Autodesk Inventor part; units mm, degrees
ref_plane "rail25_to_dummy_XY" through (0, 0, 320) normal (0, 0, 1) x (1, 0, 0)
ref_plane "rail25_to_dummy_YZ" through (0, 0, 320) normal (1, 0, 0) x (0, 1, 0)
ref_plane "rail25_to_dummy_ZX" through (0, 0, 320) normal (0, 1, 0) x (0, 0, 1)
sketch "Sketch_1" plane through (0, 0, 0) normal (0, 0, 1) x (1, 0, 0)
  arc A0 (-12.5, 1) -> (-11.5, 0) centre (-11.5, 1) ccw
  line L0 (-11.5, 0) -> (11.5, 0)
  arc A1 (11.5, 0) -> (12.5, 1) centre (11.5, 1) ccw
  line L1 (12.5, 1) -> (12.5, 7.5)
  arc A2 (12.5, 7.5) -> (11.5, 8.5) centre (11.5, 7.5) ccw
  line L2 (11.5, 8.5) -> (9.5, 8.5)
  arc A3 (9.5, 8.5) -> (8.6036, 7.9432) centre (9.5, 7.5) ccw
  arc A4 (8.5, 3.4087) -> (8.6036, 7.9432) centre (7.5, 5.7) ccw
  line L3 (8.5, 3.4087) -> (8.5, 2.5)
  arc A5 (8, 2) -> (8.5, 2.5) centre (8, 2.5) ccw
  line L4 (8, 2) -> (-8, 2)
  arc A6 (-8.5, 2.5) -> (-8, 2) centre (-8, 2.5) ccw
  line L5 (-8.5, 2.5) -> (-8.5, 3.4087)
  arc A7 (-8.6036, 7.9432) -> (-8.5, 3.4087) centre (-7.5, 5.7) ccw
  arc A8 (-8.6036, 7.9432) -> (-9.5, 8.5) centre (-9.5, 7.5) ccw
  line L6 (-9.5, 8.5) -> (-11.5, 8.5)
  arc A9 (-11.5, 8.5) -> (-12.5, 7.5) centre (-11.5, 7.5) ccw
  line L7 (-12.5, 7.5) -> (-12.5, 1)
extrude "Extrusion1" add sketch "Sketch_1" along normal blind 640
sketch "Sketch_2" plane through (0, 0, 40) normal (0, 0, 1) x (1, 0, 0)
  line L0 (0, 0) -> (0, 2)
  line L1 (0, 2) -> (4.25, 2)
  line L2 (4.25, 2) -> (2.25, 0)
  line L3 (2.25, 0) -> (0, 0)
  line L4 (0, 0) -> (0, 2)
revolve "Revolution1" cut sketch "Sketch_2" angle 360 about axis through (0, 0, 40) along (0, -1, 0)
pattern_linear "Rectangular Pattern1" count 8 spacing 80 along (0, 0, 1) of "Revolution1"
sketch "Sketch_4" plane through (0, 2, 0) normal (0, 1, 0) x (1, 0, 0)
  circle A0 centre (0, -3) radius 5
extrude "Extrusion2" add sketch "Sketch_4" along normal blind 5
sketch "Sketch_5" plane through (0, 2, 0) normal (0, 1, 0) x (1, 0, 0)
  circle A0 centre (0, -637) radius 5
extrude "Extrusion3" add sketch "Sketch_5" along normal blind 5
ref_plane "rail25_to_dummy_XY" through (0, 0, 320) normal (0, 0, 1) x (1, 0, 0)
ref_plane "rail25_to_dummy_YZ" through (0, 0, 320) normal (1, 0, 0) x (0, 1, 0)
ref_plane "rail25_to_dummy_ZX" through (0, 0, 320) normal (0, 1, 0) x (0, 0, 1)
ref_plane "to_slider_XY" through (0, 12, 320) normal (0, 0, 1) x (1, 0, 0)
ref_plane "to_slider_YZ" through (0, 12, 320) normal (1, 0, 0) x (0, 1, 0)
ref_plane "to_slider_ZX" through (0, 12, 320) normal (0, 1, 0) x (0, 0, 1)
properties part number "RSRR25-640"
For this review, take the finished solid that the model builds, in its own axes (mm). A direction names the side the tool comes from. Round coordinates to 2 decimals unless told otherwise and drop trailing zeros. Write each loop counter-clockwise with the first axis right and the second up, starting at its lowest first coordinate (ties: lowest second). Pieces come first, ordered by that corner, then holes. Notation, with made-up numbers: (19, 80.5) -> (44, 80.5) arc R15 cw to (44, 101.5) -> close; hole circle Ø7 at (-15.75, 37.25). An arc over 180 degrees is marked (long way). One line per question, with ' | ' between items. Start each with the question number.
(1) For line 1 along X through (y, z) = (6, 304); line 2 along X through (y, z) = (6.25, 567); line 3 along Z through (x, y) = (0.5, 6.5), list the stretches that pass through material, from the lowest coordinate up. Write a range as from..to.
(2) Mouldability with a two-part tool opening along X and no side actions: class faces 1 (the face through (2.307, 4.465, 632.564)), 2 (the face through (0, 0, 316)) as released by +X, released by -X, zero draft, split by the parting line, or undercut.
(3) Insertion check: P1, Ø8, axis at x = -4, z = 262.5, coming from the +Y side; P2, Ø1, axis at x = 0.5, z = 641.5, coming from the -Y side; P3, Ø8, axis at x = 0, z = 636.5, coming from the +Y side. Each pin has a flat end and moves straight along its axis. Give the tip position at first contact, or say it passes through.
(4) Tool access review of faces 3 (the face through (0, 2, 316)), 4 (the face through (0, 7, 637)): name each direction out of +Z, -Z, +X, -X, +Y, -Y from which nothing blocks a thin tool from reaching the whole face with its end or side.
(5) Add section A-A, the plane y = 5.25. Write out the cut boundary in (x, z).
(6) Add section B-B, the plane z = 429. Write out the cut boundary in (x, y).
Answer list:
1) line 1: -12.5..-9.98, 9.98..12.5 | line 2: -12.5..-9.94, 9.94..12.5 | line 3: -1.97..7.97, 632.03..641.97
2) face 1: undercut | face 2: zero draft
3) P1: y = 2 | P2: y = 2 | P3: y = 7
4) face 3: +Y | face 4: +Z, -Z, +Y
5) outline: (-12.5, 0) -> (-9.96, 0) -> (-9.96, 640) -> (-12.5, 640) -> close; circle Ø10 at (0, 3); circle Ø10 at (0, 637); (9.96, 0) -> (12.5, 0) -> (12.5, 640) -> (9.96, 640) -> close
6) outline: (-12.5, 1) arc R1 ccw to (-11.5, 0) -> (11.5, 0) arc R1 ccw to (12.5, 1) -> (12.5, 7.5) arc R1 ccw to (11.5, 8.5) -> (9.5, 8.5) arc R1 ccw to (8.6, 7.94) arc R2.5 cw to (8.5, 3.41) -> (8.5, 2.5) arc R0.5 cw to (8, 2) -> (-8, 2) arc R0.5 cw to (-8.5, 2.5) -> (-8.5, 3.41) arc R2.5 cw to (-8.6, 7.94) arc R1 ccw to (-9.5, 8.5) -> (-11.5, 8.5) arc R1 ccw to (-12.5, 7.5) -> close
